Geometry: see drawing. Coordinates: mm, zero at the bounding-box minimum. Coordinates: 2 decimals unless noted, no trailing zeros. Loops run counter-clockwise (first coordinate to the right, second up) from the corner with the lowest first, then second, coordinate; pieces in that order, holes last.
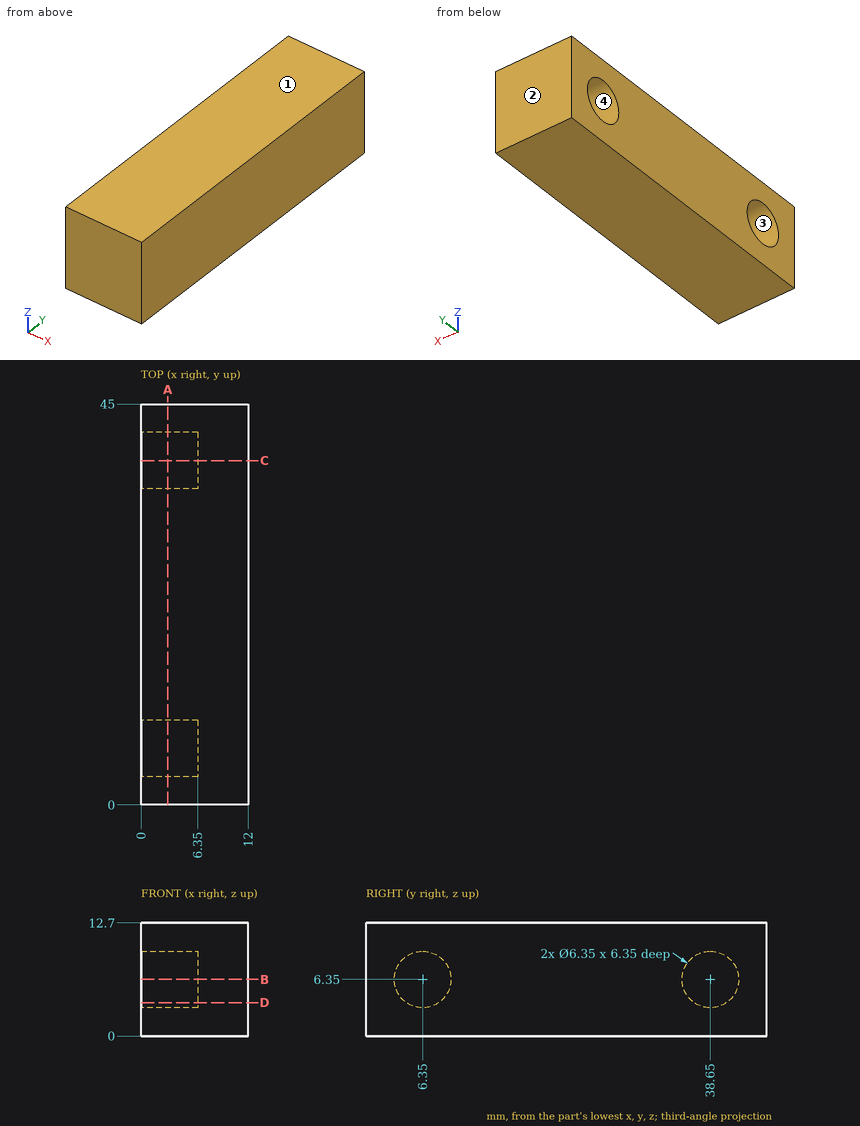
Item 1: Mould query, pull axis Y, two halves, no side actions, for the marked faces 1, 2, 3 and 4. Classes: +Y half, -Y half, draft (parallel to the pull), parting line (faces both ways), or undercut.
Result:
face 1: draft
face 2: +Y half
face 3: undercut
face 4: undercut
Item 2: Section query C-C (y = 38.65). Output: boundary loops of the cut face in (x, z) (3 decimals), then the cut area to 3 significant figures.
Result:
outline: (0, 0) - (12, 0) - (12, 12.7) - (0, 12.7) - (0, 9.525) - (6.35, 9.525) - (6.35, 3.175) - (0, 3.175) - close
area: 112 mm2
Item 3: Section query D-D (z = 3.75). Output: boundary loops of the cut face in (x, y).
Result:
outline: (0, 0) - (12, 0) - (12, 45) - (0, 45) - (0, 40.47) - (6.35, 40.47) - (6.35, 36.83) - (0, 36.83) - (0, 8.17) - (6.35, 8.17) - (6.35, 4.53) - (0, 4.53) - close
Item 4: Section query B-B (z = 6.35). Output: boundary loops of the cut face in (x, y) (3 decimals), then the cut area to 3 significant figures.
Result:
outline: (0, 0) - (12, 0) - (12, 45) - (0, 45) - (0, 41.825) - (6.35, 41.825) - (6.35, 35.475) - (0, 35.475) - (0, 9.525) - (6.35, 9.525) - (6.35, 3.175) - (0, 3.175) - close
area: 459 mm2
Item 5: Line query: L1, parallel to Y at x = 1.5, z = 6.35 (3 decimals); L2, parallel to Y at x = 5, z = 8; L3, parallel to Z at x = 5.75, y = 5. Output: solid intervals per line, ascending.
Result:
L1: y = 0 to 3.175, 9.525 to 35.475, 41.825 to 45
L2: y = 0 to 3.64, 9.06 to 35.94, 41.36 to 45
L3: z = 0 to 3.48, 9.22 to 12.7
Item 6: Section query A-A (x = 3). Output: boundary loops of the cut face in (y, z) (3 decimals).
Result:
outline: (0, 0) - (45, 0) - (45, 12.7) - (0, 12.7) - close; hole circle Ø6.35 at (6.35, 6.35); hole circle Ø6.35 at (38.65, 6.35)
